Geometry check sheet. Reference: the model listing, model coordinates, mm. Coordinates: 2 decimals unless noted, no trailing zeros. Order: outer loops, then holes, each group sorted by start corner. A loop starts at its lowest first (then second) coordinate and runs counter-clockwise, first axis right, second up. Notation, with made-up numbers: M -28,-34 L 6,-34 A19 cw 6,-20 Z; hole C 11,35.5 d5. An arc over 180 degrees is marked long. Use CSV: the item, a comma, the result in double quotes. Start each with the question number.
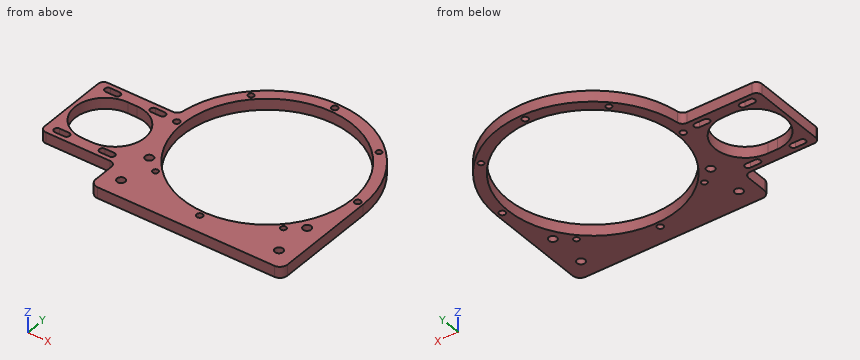
```python
from build123d import *

# Parameters (mm, degrees)
SKETCH1_R           = 2.15
SKETCH1_R_2         = 1.5
SKETCH1_R_3         = 1.65
SKETCH1_R_4         = 44.958
BOSS_EXTRUDE1_DEPTH = 5.842
FILLET1_R           = 4
BOSS_EXTRUDE2_DEPTH = 5.842
FILLET2_R           = 3


with BuildPart() as part:
    # Sketch1 → Boss-Extrude1 (new body)
    # profile 1 of 2: a face of its own
    with BuildSketch(Plane.XY):
        with BuildLine():
            ThreePointArc((50.8, 0), (0, 50.8), (-50.8, 0))
            Line((-50.8, 0), (-50.8, -57.658))
            Line((-50.8, -57.658), (0, -57.658))
            Line((0, -57.658), (50.8, -57.658))
            Line((50.8, -57.658), (50.8, 0))
        make_face()
        with Locations((-41.8, -47.658)):
            Circle(SKETCH1_R, mode=Mode.SUBTRACT)
        with Locations((-33.855565576, -33.855565576)):
            Circle(SKETCH1_R_2, mode=Mode.SUBTRACT)
        with Locations((-41.8, -27.658)):
            Circle(SKETCH1_R, mode=Mode.SUBTRACT)
        with Locations((0, -47.879)):
            Circle(SKETCH1_R_3, mode=Mode.SUBTRACT)
        with Locations((41.8, -47.658)):
            Circle(SKETCH1_R, mode=Mode.SUBTRACT)
        with Locations((33.855565576, -33.855565576)):
            Circle(SKETCH1_R_2, mode=Mode.SUBTRACT)
        with Locations((41.8, -27.658)):
            Circle(SKETCH1_R, mode=Mode.SUBTRACT)
        with Locations((-47.879, 0)):
            Circle(SKETCH1_R_3, mode=Mode.SUBTRACT)
        Circle(SKETCH1_R_4, mode=Mode.SUBTRACT)
        with Locations((-33.855565576, 33.855565576)):
            Circle(SKETCH1_R_2, mode=Mode.SUBTRACT)
        with Locations((0, 47.879)):
            Circle(SKETCH1_R_3, mode=Mode.SUBTRACT)
        with Locations((47.879, 0)):
            Circle(SKETCH1_R_3, mode=Mode.SUBTRACT)
        with Locations((33.855565576, 33.855565576)):
            Circle(SKETCH1_R_2, mode=Mode.SUBTRACT)
    # profile 2 of 2: a face of its own
    with BuildSketch(Plane.XY):
        with BuildLine():
            ThreePointArc((50.8, 0), (0, 50.8), (-50.8, 0))
            Line((-50.8, 0), (-50.8, -57.658))
            Line((-50.8, -57.658), (0, -57.658))
            Line((0, -57.658), (50.8, -57.658))
            Line((50.8, -57.658), (50.8, 0))
        make_face()
        with Locations((-41.8, -47.658)):
            Circle(SKETCH1_R, mode=Mode.SUBTRACT)
        with Locations((-33.855565576, -33.855565576)):
            Circle(SKETCH1_R_2, mode=Mode.SUBTRACT)
        with Locations((-41.8, -27.658)):
            Circle(SKETCH1_R, mode=Mode.SUBTRACT)
        with Locations((0, -47.879)):
            Circle(SKETCH1_R_3, mode=Mode.SUBTRACT)
        with Locations((41.8, -47.658)):
            Circle(SKETCH1_R, mode=Mode.SUBTRACT)
        with Locations((33.855565576, -33.855565576)):
            Circle(SKETCH1_R_2, mode=Mode.SUBTRACT)
        with Locations((41.8, -27.658)):
            Circle(SKETCH1_R, mode=Mode.SUBTRACT)
        with Locations((-47.879, 0)):
            Circle(SKETCH1_R_3, mode=Mode.SUBTRACT)
        Circle(SKETCH1_R_4, mode=Mode.SUBTRACT)
        with Locations((-33.855565576, 33.855565576)):
            Circle(SKETCH1_R_2, mode=Mode.SUBTRACT)
        with Locations((0, 47.879)):
            Circle(SKETCH1_R_3, mode=Mode.SUBTRACT)
        with Locations((47.879, 0)):
            Circle(SKETCH1_R_3, mode=Mode.SUBTRACT)
        with Locations((33.855565576, 33.855565576)):
            Circle(SKETCH1_R_2, mode=Mode.SUBTRACT)
    extrude(amount=BOSS_EXTRUDE1_DEPTH)

    # Fillet1
    fillet1_edges = [part.edges().sort_by_distance(p)[0] for p in [
        (50.8, -57.658, 2.921),
        (-50.8, -57.658, 2.921),
    ]]
    fillet(fillet1_edges, radius=FILLET1_R)

    # Sketch2 → Boss-Extrude2 (add, through all)
    with BuildSketch(Plane.XY.offset(5.842)):
        Polygon((-50.8, -39.411490459), (-50.592347052, 4.588509541), (-90.8, 4.588509541), (-90.8, -39.411490459), align=None)
        with BuildLine():
            ThreePointArc((-79.8, -33.761490459), (-78.15, -35.411490459), (-79.8, -37.061490459))
            Line((-79.8, -37.061490459), (-84.8, -37.061490459))
            ThreePointArc((-84.8, -37.061490459), (-86.45, -35.411490459), (-84.8, -33.761490459))
            Line((-84.8, -33.761490459), (-79.8, -33.761490459))
        make_face(mode=Mode.SUBTRACT)
        with BuildLine():
            ThreePointArc((-55.8, -33.761490459), (-54.15, -35.411490459), (-55.8, -37.061490459))
            Line((-55.8, -37.061490459), (-60.8, -37.061490459))
            ThreePointArc((-60.8, -37.061490459), (-62.45, -35.411490459), (-60.8, -33.761490459))
            Line((-60.8, -33.761490459), (-55.8, -33.761490459))
        make_face(mode=Mode.SUBTRACT)
        with BuildLine():
            ThreePointArc((-79.8, 2.238509541), (-78.15, 0.588509541), (-79.8, -1.061490459))
            Line((-79.8, -1.061490459), (-84.8, -1.061490459))
            ThreePointArc((-84.8, -1.061490459), (-86.45, 0.588509541), (-84.8, 2.238509541))
            Line((-84.8, 2.238509541), (-79.8, 2.238509541))
        make_face(mode=Mode.SUBTRACT)
        with BuildLine():
            ThreePointArc((-67.8, -1.411490459), (-51.8, -17.411490459), (-67.8, -33.411490459))
            Line((-67.8, -33.411490459), (-72.8, -33.411490459))
            ThreePointArc((-72.8, -33.411490459), (-88.8, -17.411490459), (-72.8, -1.411490459))
            Line((-72.8, -1.411490459), (-67.8, -1.411490459))
        make_face(mode=Mode.SUBTRACT)
        with BuildLine():
            ThreePointArc((-55.8, 2.238509541), (-54.15, 0.588509541), (-55.8, -1.061490459))
            Line((-55.8, -1.061490459), (-60.8, -1.061490459))
            ThreePointArc((-60.8, -1.061490459), (-62.45, 0.588509541), (-60.8, 2.238509541))
            Line((-60.8, 2.238509541), (-55.8, 2.238509541))
        make_face(mode=Mode.SUBTRACT)
    extrude(amount=-BOSS_EXTRUDE2_DEPTH)

    # Fillet2
    fillet2_edges = [part.edges().sort_by_distance(p)[0] for p in [
        (-50.592347052, 4.588509541, 2.921),
        (-50.8, -39.411490459, 2.921),
        (-90.8, -39.411490459, 2.921),
        (-90.8, 4.588509541, 2.921),
    ]]
    fillet(fillet2_edges, radius=FILLET2_R)


solid = part.part
```
1) Section check A-A on x = 41.8. Record the boundary of the cut face in (y, z), then the cut area to 3 significant figures.
2) Section check D-D on y = 22.5. Record the boundary of the cut face in (x, z), then the cut area to 3 significant figures.
3) Section check B-B on y = -18. Record the boundary of the cut face in (x, z).
4) Section check C-C on x = 9.5. Record the boundary of the cut face in (y, z), then the cut area to 3 significant figures.
5) Gauge pin test, flat ends, axial feed: P1, Ø1.5, axis at x = -83, z = 3, coming from the -Y side; P2, Ø1.8, axis at x = 33.86, y = -33.86, coming from the -Z side; P3, Ø1.5, axis at x = -83, z = 3.5, coming from the +Y side; P4, Ø3, axis at x = 3.5, z = 2.5, coming from the +Y side. Record the tip position at first contact, or that the pin passes through.
6) Material ranges on line 1 along Y through (x, z) = (0, 3.1); line 2 along Y through (x, z) = (1, 3.45); line 3 along X through (y, z) = (-11, 3.2), recorded low to high.
Results are:
1,outline,"M -57.66,0 L -49.81,0 L -49.81,5.84 L -57.66,5.84 Z; M -45.51,0 L -29.81,0 L -29.81,5.84 L -45.51,5.84 Z; M -25.51,0 L -16.55,0 L -16.55,5.84 L -25.51,5.84 Z; M 16.55,0 L 28.87,0 L 28.87,5.84 L 16.55,5.84 Z"
1,area,"262 mm²"
2,outline,"M -45.55,0 L -38.92,0 L -38.92,5.84 L -45.55,5.84 Z; M 38.92,0 L 45.55,0 L 45.55,5.84 L 38.92,5.84 Z"
2,area,"77.4 mm²"
3,outline,"M -90.8,0 L -88.79,0 L -88.79,5.84 L -90.8,5.84 Z; M -51.81,0 L -41.2,0 L -41.2,5.84 L -51.81,5.84 Z; M 41.2,0 L 50.8,0 L 50.8,5.84 L 41.2,5.84 Z"
4,outline,"M -57.66,0 L -43.94,0 L -43.94,5.84 L -57.66,5.84 Z; M 43.94,0 L 49.9,0 L 49.9,5.84 L 43.94,5.84 Z"
4,area,"115 mm²"
5,P1,"stops at y = -39.41"
5,P2,"passes through"
5,P3,"stops at y = 4.59"
5,P4,"stops at y = 50.76"
6,line 1,"y = -57.66 to -49.53, -46.23 to -44.96, 44.96 to 46.23, 49.53 to 50.8"
6,line 2,"y = -57.66 to -49.19, -46.57 to -44.95, 44.95 to 46.57, 49.19 to 50.79"
6,line 3,"x = -90.8 to -87.46, -53.14 to -43.59, 43.59 to 50.8"
